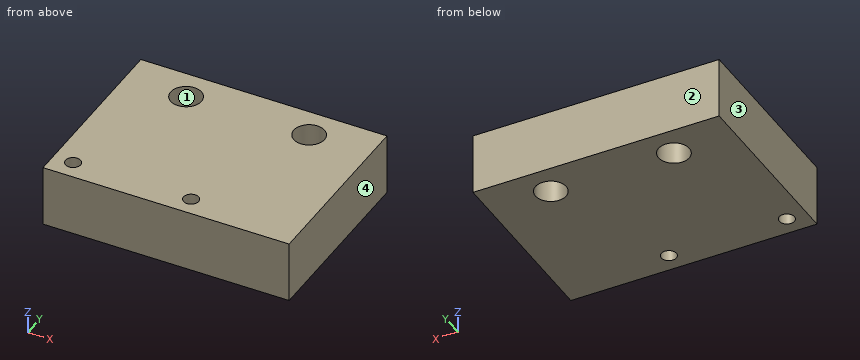
Autodesk Inventor part; units mm, degrees
ref_plane "YZ Plane" through (0, 0, 0) normal (1, 0, 0) x (0, 1, 0)
ref_plane "XZ Plane" through (0, 0, 0) normal (0, 1, 0) x (-1, 0, 0)
ref_plane "XY Plane" through (0, 0, 0) normal (0, 0, 1) x (1, 0, 0)
sketch "Sketch1" plane through (0, 0, 0) normal (0, 0, 1) x (1, 0, 0)
  line L0 (-20, 15) -> (20, 15)
  line L1 (20, 15) -> (20, -15)
  line L2 (20, -15) -> (-20, -15)
  line L3 (-20, -15) -> (-20, 15)
  point P0 (0, 0)
  point P1 (0, 15)
  point P2 (-20, 0)
  dimension "d0" = 40
  dimension "d1" = 30
extrude "Extrusion1" add sketch "Sketch1" along normal blind 10
sketch "Sketch2" plane through (0, 0, 10) normal (0, 0, 1) x (1, 0, 0)
  line L0 (20, 15) -> (-20, 15)
  line L1 (20, -15) -> (20, 15)
  line L2 (-20, 15) -> (-20, -15)
  point P0 (0, 0)
  point P1 (10, 10)
  point P2 (-10, 10)
  dimension "d4" = 5
  dimension "d5" = 10
  dimension "d6" = 10
hole "Hole1" at (10, 10, 10) at (-10, 10, 10) direction (0, 0, -1) diameter 5 end through all
sketch "Sketch3" plane through (0, 0, 10) normal (0, 0, 1) x (1, 0, 0)
  circle A0 centre (2.4125, -11.8725) radius 1.7875
  circle A1 centre (-16.7625, -11.8725) radius 1.7875
  point P0 (0, 0)
hole "Hole2" at (2.4125, -11.8725, 10) at (-16.7625, -11.8725, 10) direction (0, 0, -1) diameter 2.459 end through all
properties part number "0008-10-056"
Geometry check sheet. Reference: the model listing, model coordinates, mm. Face numbers are marked on the shaded views. Round coordinates to 2 decimals unless told otherwise and drop trailing zeros. Loops run counter-clockwise (first coordinate to the right, second up) from the corner with the lowest first, then second, coordinate; pieces in that order, holes last. Notation, with made-up numbers: (-8, 29.25) - (31, 29.25) arc R23 cw to (31, 58.25) - close; hole circle Ø8 at (87.5, 17.5). An arc over 180 degrees is marked (long way). Use a Markdown table: item, result.
Q1. Go/stop test with a flat-tipped pin: P1, Ø3, axis at x = 2.41, y = -11.87, coming from the +Z side. Record where the tip stops, or that it passes through.
Solutions:
| item | result |
|---|---|
| P1 | stops at z = 10 |
Q2. Cross-section at A-A on x = -10. Record the cut outline in (y, z).
Solutions:
| item | result |
|---|---|
| outline | (-15, 0) - (7.5, 0) - (7.5, 10) - (-15, 10) - close; (12.5, 0) - (15, 0) - (15, 10) - (12.5, 10) - close |
Q3. Draft check along X on the marked faces 1, 2, 3 and 4. Enter one of: released by +X, released by -X, zero draft, split by the parting line, or undercut.
Solutions:
| item | result |
|---|---|
| face 1 | undercut |
| face 2 | zero draft |
| face 3 | released by -X |
| face 4 | released by +X |
Q4. Cross-section at B-B on y = 12. Record the cut outline in (x, z), plus the area to 3 significant figures.
Solutions:
| item | result |
|---|---|
| outline | (-20, 0) - (-11.5, 0) - (-11.5, 10) - (-20, 10) - close; (-8.5, 0) - (8.5, 0) - (8.5, 10) - (-8.5, 10) - close; (11.5, 0) - (20, 0) - (20, 10) - (11.5, 10) - close |
| area | 340 mm2 |
Q5. Cross-section at C-C on z = 9.25. Record the cut outline in (x, y).
Solutions:
| item | result |
|---|---|
| outline | (-20, -15) - (20, -15) - (20, 15) - (-20, 15) - close; hole circle Ø2.46 at (-16.76, -11.87); hole circle Ø5 at (-10, 10); hole circle Ø2.46 at (2.41, -11.87); hole circle Ø5 at (10, 10) |
Q6. Cross-section at D-D on x = -16. Record the cut outline in (y, z), plus the area to 3 significant figures.
Solutions:
| item | result |
|---|---|
| outline | (-15, 0) - (-12.84, 0) - (-12.84, 10) - (-15, 10) - close; (-10.91, 0) - (15, 0) - (15, 10) - (-10.91, 10) - close |
| area | 281 mm2 |
Q7. Material ranges on line 1 (X direction, y = 10, z = 7.75); line 2 (Y direction, x = -10, z = 4); line 3 (X direction, y = 11.75, z = 1), recorded low to high.
Solutions:
| item | result |
|---|---|
| line 1 | x = -20 to -12.5, -7.5 to 7.5, 12.5 to 20 |
| line 2 | y = -15 to 7.5, 12.5 to 15 |
| line 3 | x = -20 to -11.79, -8.21 to 8.21, 11.79 to 20 |
